```python
from build123d import *

# Parameters (mm, degrees)
F0_W     = 30
F0_H     = 20
F1_DEPTH = 15
F2_W     = 10
F2_H     = 5
F3_DEPTH = 30.001
F4_W     = 20
F4_H     = 5
F5_DEPTH = 20.001
F7_R     = 2.5
F8_DEPTH = 10.001


with BuildPart() as f1:
    # F0 (on Top) → F1 (new body)
    with BuildSketch(Plane.XY):
        with Locations((4.308961, 9.361647)):
            Rectangle(F0_W, F0_H)
    extrude(amount=F1_DEPTH)

    # F2 (on face) → F3 (cut, through all)
    with BuildSketch(Plane.YZ.offset(19.308961)):
        with Locations((9.361647, 2.5)):
            Rectangle(F2_W, F2_H)
    extrude(amount=-F3_DEPTH, mode=Mode.SUBTRACT)

    # F4 (on face) → F5 (cut, through all)
    with BuildSketch(Plane(origin=(0, 19.361647, 0), x_dir=(-1, 0, 0), z_dir=(0, 1, 0))):
        with Locations((-4.308961, 12.5)):
            Rectangle(F4_W, F4_H)
    extrude(amount=-F5_DEPTH, mode=Mode.SUBTRACT)

    # F7 (on face) → F8 (cut, through all)
    with BuildSketch(Plane.XY.offset(10)):
        with Locations((-0.683151, 9.394292)):
            Circle(F7_R)
        with Locations((9.317168, 9.394293)):
            Circle(F7_R)
    extrude(amount=-F8_DEPTH, mode=Mode.SUBTRACT)


solid = f1.part
```
Read the model definition and answer for the solid it produces. Units are mm, in the model's axes. A direction names the side the tool comes from. Give positions to 0.01 mm unless a question says otherwise; leave off trailing zeros. Order: outer loops, then holes, each group sorted by start corner. A loop starts at its lowest first (then second) coordinate and runs counter-clockwise, first axis right, second up. Notation, with made-up numbers: (49.25, -17) -> (94.25, -17) arc R22 cw to (94.25, 17) -> close; hole circle Ø11 at (-31, -7). An arc over 180 degrees is marked (long way). Write item = value, one per line.
1. A cutting plane is placed at B-B, the plane x = 13. Write down the section's boundary in (y, z).
Numbers:
outline = (-0.64, 0) -> (4.36, 0) -> (4.36, 5) -> (14.36, 5) -> (14.36, 0) -> (19.36, 0) -> (19.36, 10) -> (-0.64, 10) -> close
2. A cutting plane is placed at D-D, the plane x = 9.75. Write down the section's boundary in (y, z).
Numbers:
outline = (-0.64, 0) -> (4.36, 0) -> (4.36, 5) -> (6.93, 5) -> (6.93, 10) -> (-0.64, 10) -> close; (11.86, 5) -> (14.36, 5) -> (14.36, 0) -> (19.36, 0) -> (19.36, 10) -> (11.86, 10) -> close
3. The mould has two halves that part along Y. Classify faces 4 (the face through (-8, 10, 15)), 5 (the face through (5, 4.362, 2)), 6 (the face through (4, 19.362, 6)): +Y half, -Y half, draft (parallel to the pull), parting line (faces both ways), or undercut.
Numbers:
face_4 = draft
face_5 = undercut
face_6 = +Y half
4. For faces 1 (the face through (5, 14.362, 2)), 2 (the face through (-10.691, 9, 9)), 3 (the face through (14.309, 10, 12)), determine the directions among +Z, -Z, +X, -X, +Y, -Y from which every point of the face is accessible in a straight line to the end or side of a thin tool.
Numbers:
face_1 = -Z, +X, -X
face_2 = +Z, -Z, -X, +Y, -Y
face_3 = +Z, +Y, -Y
5. A cutting plane is placed at A-A, the plane z = 13. Write down the section's boundary in (x, y), and give its area (3 significant figures).
Numbers:
outline = (-10.69, -0.64) -> (-5.69, -0.64) -> (-5.69, 19.36) -> (-10.69, 19.36) -> close; (14.31, -0.64) -> (19.31, -0.64) -> (19.31, 19.36) -> (14.31, 19.36) -> close
area = 200 mm²
6. Straight lines are drawn through the part: line 1 along X through (y, z) = (15.25, 11); line 2 along Y through (x, z) = (-7, 2.5); line 3 along X through (y, z) = (10.25, 6.5). For each, find the intervals that lie inside material, in ascending order.
Numbers:
line_1 = -10.69 to -5.69, 14.31 to 19.31
line_2 = -0.64 to 4.36, 14.36 to 19.36
line_3 = -10.69 to -3.03, 1.67 to 6.97, 11.67 to 19.31
7. Given pin 1 (6.5 mm diameter, centred on x = 9.32, y = 9.39, fed in from +Z); pin 2 (1.5 mm diameter, centred on x = 14, y = 9, fed in from -Z), each flat-ended and moving along its own axis, determine where each tip first touches the part or whether it passes through.
Numbers:
pin_1 = 10
pin_2 = 5
8. A cutting plane is placed at C-C, the plane y = 2.25. Write down the section's boundary in (x, z), and give its area (3 significant figures).
Numbers:
outline = (-10.69, 0) -> (19.31, 0) -> (19.31, 15) -> (14.31, 15) -> (14.31, 10) -> (-5.69, 10) -> (-5.69, 15) -> (-10.69, 15) -> close
area = 350 mm²
